The listing builds one solid part. Answer for the finished solid, in the listing's coordinates (mm). A direction names the side the tool comes from. Round coordinates to 2 decimals unless told otherwise and drop trailing zeros. Loops run counter-clockwise (first coordinate to the right, second up) from the corner with the lowest first, then second, coordinate; pieces in that order, holes last. Notation, with made-up numbers: (3, 56.5) -> (50, 56.5) arc R10 cw to (50, 60.5) -> close; hole circle Ø4 at (16.5, 18.5). An arc over 180 degrees is marked (long way). Use a Markdown table: item, result. Add a question column.
Q1. Section B-B on z = 0 is taken. Give the number of separate pieces and of enclosed holes in the cut face, then the cut area to 3 significant figures.
Q2. Section A-A on x = 9 is taken. Give the vertices of the cut face in (y, z).
Q3. Given pin 1 Ø4 at (y, z) = (-1, 0) entering from -X; pin 2 Ø2 at (x, z) = (11, -1.5) entering from +Y; pin 3 Ø8 at (x, y) = (25.5, -0.5) entering from +Z; pin 4 Ø2 at (x, y) = (7, -1.5) entering from -Z, each flat-ended and moving along its own axis, determine where each tip first touches the part or whether it passes through.
Q4. Which of the six approach directions +Z, -Z, +X, -X, +Y, -Y give full straight-line access (tool end or side, diameter ignored) to faces 4 (the flat face through (0, -3, -3)), 5 (the cylindrical face through (5.93, 1.65, 5.53)), 6 (the cylindrical face through (5.93, 5.53, -1.65))?
Q5. Section D-D on z = -4.5 is taken. Give the vertices of the cut face in (x, y), then the cut area to 3 significant figures.
Q6. Consider line 1 (X direction, y = 4.8, z = 0); line 2 (Z direction, x = 25, y = 0) (3 decimals); line 3 (Z direction, x = 10.25, y = 0). Determine where each line is inside the solid, lowest interval first.
Q7. For a pull along Y with two mould halves and no side action, classify faces 1 (the cylindrical face through (14.79, -6.654, -3.461)), 2 (the cylindrical face through (7.4, -1.49, -3.58)), 3 (the flat face through (30, -3, -2)) as released by +Y, released by -Y, zero draft, split by the parting line, or undercut.
from build123d import *

# Parameters (mm, degrees)
CROQUIS1_R              = 7.5
CROQUIS1_R_2            = 3.877864762
SALIENTE_EXTRUIR1_DEPTH = 15
CROQUIS3_R              = 7.5
CROQUIS3_R_2            = 3.175
SALIENTE_EXTRUIR2_DEPTH = 15


with BuildPart() as part:
    # Croquis1 → Saliente-Extruir1 (new body)
    with BuildSketch(Plane(origin=(0, 0, 0), x_dir=(0, 0, -1), z_dir=(1, 0, 0))):
        Circle(CROQUIS1_R)
        Circle(CROQUIS1_R_2, mode=Mode.SUBTRACT)
    extrude(amount=SALIENTE_EXTRUIR1_DEPTH)

    # Croquis3 → Saliente-Extruir2 (add)
    with BuildSketch(Plane(origin=(15, 0, 0), x_dir=(0, 0, -1), z_dir=(1, 0, 0))):
        Circle(CROQUIS3_R)
        Circle(CROQUIS3_R_2, mode=Mode.SUBTRACT)
    extrude(amount=SALIENTE_EXTRUIR2_DEPTH)

    # Croquis5 → Perforador para roscar para macho de roscar para M4x0.72 (revolve, cut)
    with BuildSketch(Plane(origin=(6, 7.5, 0), x_dir=(0, 0, 1), z_dir=(1, 0, 0))):
        Polygon((0, 0), (0, 8.491420021), (1.65, 7.5), (1.65, 0), align=None)
    revolve(axis=Axis((6, 13.85, 0), (0, -1, 0)), mode=Mode.SUBTRACT)

    # Croquis5 at point 2 (carried to point 2, square into its face) → Perforador para roscar para macho de 2 (revolve, cut)
    with BuildSketch(Plane(origin=(6, 0, 7.5), x_dir=(0, -1, 0), z_dir=(1, 0, 0))):
        Polygon((0, 0), (0, 8.491420021), (1.65, 7.5), (1.65, 0), align=None)
    revolve(axis=Axis((6, 0, 13.85), (0, 0, -1)), mode=Mode.SUBTRACT)

    # Croquis5 at point 3 (carried to point 3, square into its face) → Perforador para roscar para macho de 3 (revolve, cut)
    with BuildSketch(Plane(origin=(-116.474048572, 0, -29.182020138), x_dir=(0, 0, 1), z_dir=(1, 0, 0))):
        Polygon((0, 0), (0, 8.491420021), (1.65, 7.5), (1.65, 0), align=None)
    revolve(axis=Axis((-116.474048572, 6.35, -29.182020138), (0, -1, 0)), mode=Mode.SUBTRACT)

    # MatrizL1: read off the stored shape, not the designer's step
    # MatrizL1: loft between two sections, ruled curve by curve
    matrizl1_from = [
        Edge.make_three_point_arc((22.65, 0, 2.712370176), (21, 1.65, 2.712370176), (19.35, 0, 2.712370176)),
        Edge.make_three_point_arc((19.35, 0, 2.712370176), (21, -1.65, 2.712370176), (22.65, 0, 2.712370176)),
    ]
    matrizl1_to = [
        Edge.make_three_point_arc((22.65, 0, 7.500099893), (21, 1.65, 7.500099893), (19.35, 0, 7.500099893)),
        Edge.make_three_point_arc((19.35, 0, 7.500099893), (21, -1.65, 7.500099893), (22.65, 0, 7.500099893)),
    ]
    matrizl1 = Solid(Shell([*[Face.make_surface_from_curves(matrizl1_from[k], matrizl1_to[k]) for k in range(2)], Face(Wire(matrizl1_from)), Face(Wire(matrizl1_to))]))
    add(matrizl1, mode=Mode.SUBTRACT)

    # MatrizL1 2: loft between two sections, ruled curve by curve
    matrizl1_2_from = [
        Edge.make_three_point_arc((21, 2.712383518, 1.65), (22.65, 2.712383518, 0), (21, 2.712383518, -1.65)),
        Edge.make_three_point_arc((21, 2.712383518, -1.65), (19.35, 2.712383518, 0), (21, 2.712383518, 1.65)),
    ]
    matrizl1_2_to = [
        Edge.make_three_point_arc((21, 7.50002686, 1.65), (22.65, 7.50002686, 0), (21, 7.50002686, -1.65)),
        Edge.make_three_point_arc((21, 7.50002686, -1.65), (19.35, 7.50002686, 0), (21, 7.50002686, 1.65)),
    ]
    matrizl1_2 = Solid(Shell([*[Face.make_surface_from_curves(matrizl1_2_from[k], matrizl1_2_to[k]) for k in range(2)], Face(Wire(matrizl1_2_from)), Face(Wire(matrizl1_2_to))]))
    add(matrizl1_2, mode=Mode.SUBTRACT)


solid = part.part
Checked values:
| question | item | result |
|---|---|---|
| 1 | separate pieces | 4 |
| 1 | enclosed holes | 0 |
| 1 | area | 212 mm2 |
| 2 | outline | circle Ø15 at (0, 0); hole circle Ø7.76 at (0, 0) |
| 3 | pin 1 | passes through |
| 3 | pin 2 | stops at y = 7.48 |
| 3 | pin 3 | stops at z = 7.5 |
| 3 | pin 4 | stops at z = -7.48 |
| 4 | face 4 | +Z, -Z, -X, +Y, -Y |
| 4 | face 5 | +Z |
| 4 | face 6 | +Y |
| 5 | outline | (0, -6) -> (30, -6) -> (30, 6) -> (0, 6) -> close |
| 5 | area | 360 mm2 |
| 6 | line 1 | x = 0 to 4.35, 7.65 to 19.35, 22.65 to 30 |
| 6 | line 2 | z = -7.5 to -3.175, 3.175 to 7.5 |
| 6 | line 3 | z = -7.5 to -3.88, 3.88 to 7.5 |
| 7 | face 1 | split by the parting line |
| 7 | face 2 | undercut |
| 7 | face 3 | zero draft |
